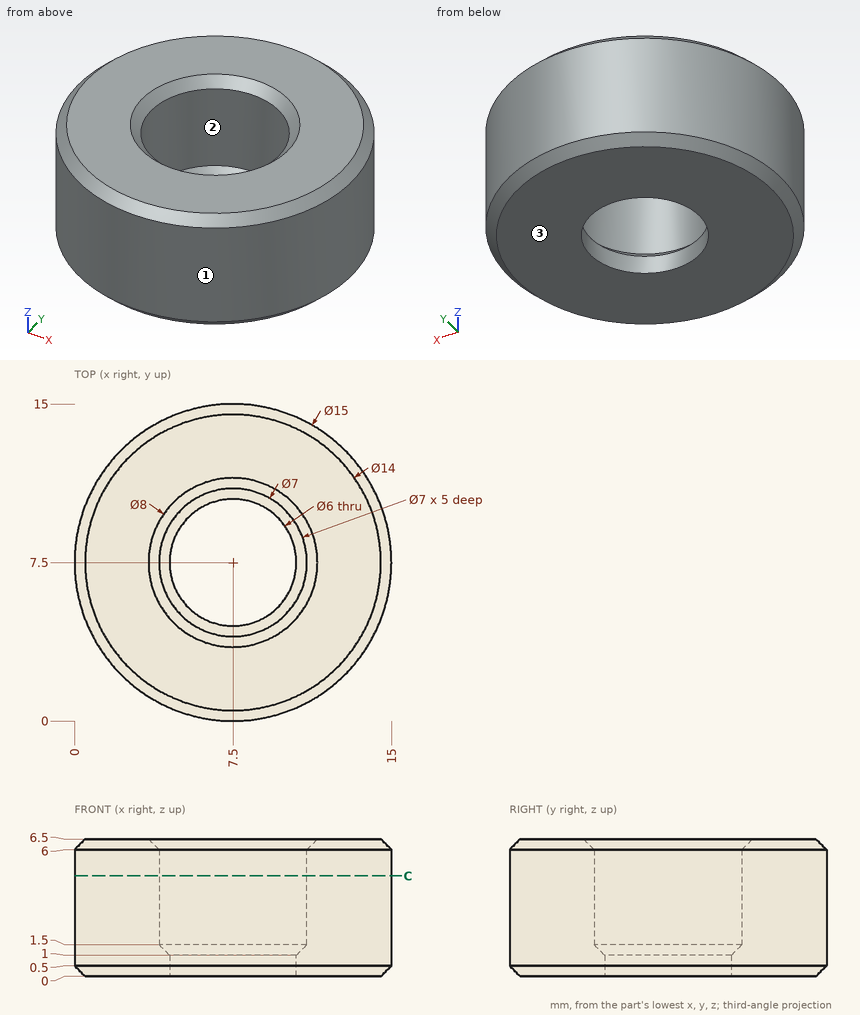
Could you check a few things on this drawing? It's one solid part, dimensions in mm from its lowest x, y, z. Coordinates: 2 decimals unless noted, no trailing zeros. Write each loop counter-clockwise with the first axis right and the second up, starting at its lowest first coordinate (ties: lowest second). Pieces come first, ordered by that corner, then holes. Notation, with made-up numbers: (-27, 75) - (9, 75) arc R30 cw to (9, 99) - close; hole circle Ø11 at (16.25, -2.75). An arc over 180 degrees is marked (long way). Return JSON: item names as keys, results as strings. Group by question number.
Item 1: Please list where these lines run through material, in increasing order: probe 1 along Y at (x, z) = (7.5, 4.75); probe 2 along X at (y, z) = (10.25, 4) (1 decimal); probe 3 along Y at (x, z) = (7.5, 0.55).
Item 2: We'd pull the mould along Y, two halves only. Please class the marked faces 1, 2 and 3: pulls with the +Y half, pulls with the -Y half, needs draft (parallel to the pull), parting line crosses it, or undercut.
Item 3: I'm going to push flat-ended pins straight in: pin 1 Ø1.5 at (y, z) = (3, 3.5) entering from -X; pin 2 Ø1 at (x, z) = (3.5, 3.5) entering from +Y; pin 3 Ø2 at (x, z) = (2, 2) entering from -Y. Where does each tip first touch, or does it pass through?
Item 4: If we section it at C-C (z = 4.75): Write out the boundary of the cut face in (x, y), then the cut area to 3 significant figures.
Return value:
{
 "1": {"probe 1": "y = 0 to 4, 11 to 15", "probe 2": "x = 0.5 to 5.3, 9.7 to 14.5", "probe 3": "y = 0 to 4.5, 10.5 to 15"},
 "2": {"face 1": "parting line crosses it", "face 2": "undercut", "face 3": "needs draft"},
 "3": {"pin 1": "stops at x = 1", "pin 2": "stops at y = 14.13", "pin 3": "stops at y = 1.5"},
 "4": {"outline": "circle Ø15 at (7.5, 7.5); hole circle Ø7 at (7.5, 7.5)", "area": "138 mm^2"}
}
